Autodesk Fusion 360 part; units mm, degrees
sketch "Sketch2" plane through (0, 0, 0) normal (0, 1, 0) x (1, 0, 0)
  line L0 (24.9, -34.9) -> (-24.9, -34.9)
  line L1 (-24.9, -34.9) -> (-24.9, 34.9)
  line L2 (-24.9, 34.9) -> (24.9, 34.9)
  line L3 (24.9, 34.9) -> (24.9, -34.9)
  line L4 (24.9, -34.9) -> (-24.9, 34.9) construction
  line L5 (-24.9, -34.9) -> (24.9, 34.9) construction
  dimension "d1" = 49.8
  dimension "d2" = 69.8
extrude "Extrude1" add sketch "Sketch2" along normal blind 2
sketch "Sketch3" plane through (0, 0, 0) normal (0, -1, 0) x (1, 0, 0)
  line L0 (-24.9, -34.9) -> (24.9, -34.9)
  line L1 (24.9, -34.9) -> (24.9, 34.9)
  line L2 (24.9, 34.9) -> (-24.9, 34.9)
  line L3 (-24.9, 34.9) -> (-24.9, -34.9)
  line L4 (15.2, 20.15) -> (-15.2, 20.15)
  line L5 (-15.2, 20.15) -> (-15.2, 5.85)
  line L6 (-15.2, 5.85) -> (15.2, 5.85)
  line L7 (15.2, 5.85) -> (15.2, 20.15)
  line L8 (15.2, 20.15) -> (-15.2, 5.85) construction
  line L9 (-15.2, 20.15) -> (15.2, 5.85) construction
  line L10 (17.85, 23.03) -> (-22.3, 23.03) construction
  line L11 (-22.3, 23.03) -> (-22.3, 2.97) construction
  line L12 (-22.3, 2.97) -> (17.85, 2.97) construction
  line L13 (17.85, 2.97) -> (17.85, 23.03) construction
  line L14 (17.85, 23.03) -> (-22.3, 2.97) construction
  line L15 (-22.3, 23.03) -> (17.85, 2.97) construction
  line L16 (0, 13) -> (15.2, 13) construction
  circle A0 centre (8.55, 23.03) radius 1.5
  circle A1 centre (8.55, 2.97) radius 1.5
  circle A2 centre (-22.3, 13) radius 1.5
  point P0 (0, 13)
  point P1 (-2.225, 13)
  dimension "d5" = 30.4
  dimension "d6" = 14.3
  dimension "d7" = 40.15
  dimension "d8" = 20.06
  dimension "d10" = 2.65
  dimension "d11" = 3
  dimension "d12" = 9.3
  dimension "d13" = 3
extrude "Extrude2" cut sketch "Sketch3" against normal blind 2 contours L4 L5 L6 L7 | A0 | A1 | A2
sketch "Sketch5" plane through (0, 2, 0) normal (0, 1, 0) x (-1, 0, 0)
  circle A0 centre (22.3, 13) radius 1.5
  circle A1 centre (-8.55, 2.97) radius 1.5
  line L0 (-15.2, 20.15) -> (15.2, 20.15)
  line L1 (15.2, 20.15) -> (15.2, 5.85)
  line L2 (15.2, 5.85) -> (-15.2, 5.85)
  line L3 (-15.2, 5.85) -> (-15.2, 20.15)
  circle A2 centre (-8.55, 23.03) radius 1.5
  line L4 (-24.9, -34.9) -> (24.9, -34.9)
  line L5 (24.9, -34.9) -> (24.9, 34.9)
  line L6 (24.9, 34.9) -> (-24.9, 34.9)
  line L7 (-24.9, 34.9) -> (-24.9, -34.9)
  line L8 (-26.9, -36.9) -> (26.9, -36.9)
  line L9 (26.9, -36.9) -> (26.9, 36.9)
  line L10 (26.9, 36.9) -> (-26.9, 36.9)
  line L11 (-26.9, 36.9) -> (-26.9, -36.9)
  line L12 (-23.9, 33.9) -> (-23.9, -33.9)
  line L13 (-23.9, -33.9) -> (23.9, -33.9)
  line L14 (23.9, -33.9) -> (23.9, 33.9)
  line L15 (23.9, 33.9) -> (-23.9, 33.9)
  line L16 (0, 34.9) -> (0, -34.9) construction
  line L17 (-24.9, 0) -> (24.9, 0) construction
  line L18 (-10, 33.9) -> (10, 33.9)
  line L19 (10, 33.9) -> (10, 36.9)
  line L20 (10, 36.9) -> (-10, 36.9)
  line L21 (-10, 36.9) -> (-10, 33.9)
  line L22 (10, -36.9) -> (-10, -36.9)
  line L23 (10, -33.9) -> (10, -36.9)
  line L24 (-10, -36.9) -> (-10, -33.9)
  line L25 (-10, -33.9) -> (10, -33.9)
  dimension "d17" = 2
  dimension "d18" = -1
  dimension "d34" = 20
  dimension "d35" = 10
extrude "Extrude3" add sketch "Sketch5" along normal blind 1 contours L4 L6 L7 L12 L13 L15 L21 L24 | L4 L6 L7 L8 L10 L11 L21 L24 | L4 L5 L6 L13 L14 L15 L19 L23 | L4 L5 L6 L8 L9 L10 L19 L23
sketch "Sketch6" plane through (0, 2, 0) normal (0, 1, 0) x (-1, 0, 0)
  line L0 (-23.9, 33.9) -> (-23.9, -33.9)
  line L1 (-23.9, -33.9) -> (-10, -33.9)
  line L2 (23.9, -33.9) -> (23.9, 33.9)
  line L3 (-10, 33.9) -> (-23.9, 33.9)
  circle A0 centre (22.3, 13) radius 1.5
  circle A1 centre (-8.55, 2.97) radius 1.5
  line L4 (-15.2, 20.15) -> (15.2, 20.15)
  line L5 (15.2, 20.15) -> (15.2, 5.85)
  line L6 (15.2, 5.85) -> (-15.2, 5.85)
  line L7 (-15.2, 5.85) -> (-15.2, 20.15)
  circle A2 centre (-8.55, 23.03) radius 1.5
  circle A3 centre (22.3, 13) radius 3
  line L8 (10, 33.9) -> (10, 34.9)
  line L9 (10, 34.9) -> (-10, 34.9)
  line L10 (-10, 34.9) -> (-10, 33.9)
  line L11 (-10, -33.9) -> (-10, -34.9)
  line L12 (-10, -34.9) -> (10, -34.9)
  line L13 (10, -34.9) -> (10, -33.9)
  line L14 (10, -33.9) -> (23.9, -33.9)
  line L15 (23.9, 33.9) -> (10, 33.9)
  dimension "d21" = 6
extrude "Extrude4" cut sketch "Sketch6" along normal blind 1 contours L2 A3 | L2 A3
sketch "Sketch9" plane through (0, 2, 0) normal (0, 1, 0) x (-1, 0, 0)
  circle A0 centre (22.3, 13) radius 1.5
  line L0 (23.9, 15.5377) -> (23.9, 33.9)
  line L1 (23.9, 33.9) -> (10, 33.9)
  line L2 (10, 33.9) -> (10, 34.9)
  line L3 (10, 34.9) -> (-10, 34.9)
  line L4 (-10, 34.9) -> (-10, 33.9)
  line L5 (-10, 33.9) -> (-23.9, 33.9)
  line L6 (-23.9, 33.9) -> (-23.9, -33.9)
  line L7 (-23.9, -33.9) -> (-10, -33.9)
  line L8 (-10, -33.9) -> (-10, -34.9)
  line L9 (-10, -34.9) -> (10, -34.9)
  line L10 (10, -34.9) -> (10, -33.9)
  line L11 (10, -33.9) -> (23.9, -33.9)
  line L12 (23.9, -33.9) -> (23.9, 10.4623)
  arc A1 (23.9, 10.4623) -> (24.9, 11.5033) centre (22.3, 13) ccw
  line L13 (24.9, 11.5033) -> (24.9, 14.4967)
  arc A2 (24.9, 14.4967) -> (23.9, 15.5377) centre (22.3, 13) ccw
  circle A3 centre (-8.55, 23.03) radius 1.5
  line L14 (-15.2, 20.15) -> (15.2, 20.15)
  line L15 (15.2, 20.15) -> (15.2, 5.85)
  line L16 (15.2, 5.85) -> (-15.2, 5.85)
  line L17 (-15.2, 5.85) -> (-15.2, 20.15)
  circle A4 centre (-8.55, 2.97) radius 1.5
  line L18 (0, 34.9) -> (0, -34.9) construction
  line L19 (-27, 0) -> (27, 0) construction
  line L20 (-4.5, 34.9) -> (4.5, 34.9)
  line L21 (4.5, 34.9) -> (4.5, 31.9)
  line L22 (4.5, 31.9) -> (-4.5, 31.9)
  line L23 (-4.5, 31.9) -> (-4.5, 34.9)
  line L24 (-4.5, -34.9) -> (4.5, -34.9)
  line L25 (-4.5, -31.9) -> (-4.5, -34.9)
  line L26 (4.5, -31.9) -> (-4.5, -31.9)
  line L27 (4.5, -34.9) -> (4.5, -31.9)
  dimension "d36" = 9
  dimension "d37" = 3
  dimension "d38" = 4.5
extrude "Extrude7" add sketch "Sketch9" along normal blind 9 contours L3 L20 L21 L22 L23 | L9 L24 L25 L26 L27
sketch "Sketch10" plane through (0, 0, -34.9) normal (0, 0, -1) x (1, 0, 0)
  line L0 (24.9, 0) -> (-24.9, 0)
  line L1 (-24.9, 0) -> (-24.9, -2)
  line L2 (-24.9, -2) -> (-10, -2)
  line L3 (-10, -2) -> (-4.5, -2)
  line L4 (-4.5, -2) -> (-4.5, -11)
  line L5 (-4.5, -11) -> (4.5, -11)
  line L6 (4.5, -11) -> (4.5, -2)
  line L7 (4.5, -2) -> (10, -2)
  line L8 (10, -2) -> (24.9, -2)
  line L9 (24.9, -2) -> (24.9, 0)
  line L10 (-4.5, -2) -> (4.5, -11) construction
  line L11 (4.5, -2) -> (-4.5, -11) construction
  circle A0 centre (0, -6.5) radius 2.15
  dimension "d41" = 4.3
extrude "Extrude8" cut sketch "Sketch10" against normal blind 72 contours A0
fillet "Fillet2" radius 4.5 8 edges at (4.5, 2, 33.4) (4.5, 11, 33.4) (-4.5, 11, 33.4) (-4.5, 2, 33.4) (-4.5, 11, -33.4) (-4.5, 2, -33.4) (4.5, 2, -33.4) (4.5, 11, -33.4)
Input: part model. Units: mm. Frame: model coordinates. A direction names the side the tool comes from. Give positions to 0.01 mm unless a question says otherwise; leave off trailing zeros. Order: outer loops, then holes, each group sorted by start corner. A loop starts at its lowest first (then second) coordinate and runs counter-clockwise, first axis right, second up. Notation, with made-up numbers: (87, 4.5) - (110, 4.5) arc R21 ccw to (110, 8.5) - close; hole circle Ø7 at (75.5, 10.25). An arc over 180 degrees is marked (long way). Use a Markdown table: item, result.
(1) Draft query along Z for faces 1 (the cylindrical face through (3.217, 9.647, 33.421)), 2 (the flat face through (0, 3, 34.9)), 3 (the flat face through (2, 5, 31.9)). Return one class per face: released by +Z, released by -Z, zero draft, split by the parting line, or undercut.
Computed values:
| item | result |
|---|---|
| face 1 | zero draft |
| face 2 | released by +Z |
| face 3 | undercut |
(2) Pin query (flat end, axial travel): pin 1 (0.6 mm diameter, centred on x = 2.5, y = 1, fed in from +Z); pin 2 (12 mm diameter, centred on x = -18, z = 20, fed in from +Y); pin 3 (12 mm diameter, centred on x = -4.5, z = 17, fed in from +Y); pin 4 (2.5 mm diameter, centred on x = 8.55, z = 2.97, fed in from +Y). Return the tip coordinate at first contact, or that it passes through.
Computed values:
| item | result |
|---|---|
| pin 1 | stops at z = 34.9 |
| pin 2 | stops at y = 3 |
| pin 3 | stops at y = 2 |
| pin 4 | passes through |
(3) Section query D-D (z = 13). Output: boundary loops of the cut face in (x, y), then the cut area to 3 significant figures.
Computed values:
| item | result |
|---|---|
| outline | (-26.9, 2) - (-25.3, 2) - (-25.3, 3) - (-26.9, 3) - close; (-24.9, 0) - (-23.8, 0) - (-23.8, 2) - (-24.9, 2) - close; (-20.8, 0) - (-15.2, 0) - (-15.2, 2) - (-20.8, 2) - close; (15.2, 0) - (24.9, 0) - (24.9, 2) - (26.9, 2) - (26.9, 3) - (23.9, 3) - (23.9, 2) - (15.2, 2) - close |
| area | 37.4 mm2 |
(4) Section query B-B (z = 23.03). Output: boundary loops of the cut face in (x, y).
Computed values:
| item | result |
|---|---|
| outline | (-26.9, 2) - (-24.9, 2) - (-24.9, 0) - (7.05, 0) - (7.05, 2) - (-23.9, 2) - (-23.9, 3) - (-26.9, 3) - close; (10.05, 0) - (24.9, 0) - (24.9, 2) - (26.9, 2) - (26.9, 3) - (23.9, 3) - (23.9, 2) - (10.05, 2) - close |
(5) Section query A-A (x = -22.3). Output: boundary loops of the cut face in (y, z).
Computed values:
| item | result |
|---|---|
| outline | (0, -34.9) - (2, -34.9) - (2, -36.9) - (3, -36.9) - (3, -33.9) - (2, -33.9) - (2, 11.5) - (0, 11.5) - close; (0, 14.5) - (2, 14.5) - (2, 33.9) - (3, 33.9) - (3, 36.9) - (2, 36.9) - (2, 34.9) - (0, 34.9) - close |
(6) Line query: line 1 (X direction, y = 2.75, z = -15); line 2 (Z direction, x = -6, y = 2.5); line 3 (X direction, y = 6.5, z = -33.15). Output: solid intervals per line, ascending. Write a range as from..to.
Computed values:
| item | result |
|---|---|
| line 1 | x = -26.9..-23.9, 23.9..26.9 |
| line 2 | z = -34.9..-31.9, 31.9..34.9 |
| line 3 | x = -4.5..-2.15, 2.15..4.5 |
(7) Section query C-C (y = 1). Output: boundary loops of the cut face in (x, z), then the cut area to 3 significant figures.
Computed values:
| item | result |
|---|---|
| outline | (-24.9, -34.9) - (24.9, -34.9) - (24.9, 34.9) - (-24.9, 34.9) - close; hole circle Ø3 at (-22.3, 13); hole (-15.2, 5.85) - (15.2, 5.85) - (15.2, 20.15) - (-15.2, 20.15) - close; hole circle Ø3 at (8.55, 2.97); hole circle Ø3 at (8.55, 23.03) |
| area | 3,020 mm2 |
(8) Access query for faces 4 (the flat face through (0, 1, 5.85)), 5 (the cylindrical face through (5.783, 3.353, 33.421)), 6 (the cylindrical face through (-2.15, 6.41, 33.38)), 7 (the flat face through (2, 5, -31.9)). Directions: +Z, -Z, +X, -X, +Y, -Y. A direction counts if a zero-diameter tool reaches every point of the face in a straight line with its end or side. Return the directions, or none.
Computed values:
| item | result |
|---|---|
| face 4 | +Y, -Y |
| face 5 | +Z, -Z, +Y |
| face 6 | +Z, -Z |
| face 7 | +Y |
